Can you work these out from the drawing? Everything is in mm from the part's minimum corner. Give positions to 0.01 mm unless a question says otherwise; leave off trailing zeros. Order: outer loops, then holes, each group sorted by start corner. A loop starts at its lowest first (then second) coordinate and runs counter-clockwise, first axis right, second up. Notation, with made-up numbers: M 86.5,66.25 L 140.5,66.25 A36 cw 140.5,100.25 Z; hole C 53,9.25 d8. An arc over 180 degrees is marked long. Use a Markdown table: item, result. Add a question column.
Item 1: Suppose I cut it at B-B on z = 0.6. Count the separate pieces of the cut face and the enclosed holes in it, plus the area to 3 significant figures.
Item 2: If I drill on L1, parallel to Y at x = 25, z = 2.25; L2, parallel to Z at x = 12, y = 31.75; L3, parallel to Y at x = 17.5, z = 4.45, over which ranges is the centre line in solid material (lowest first)? Write a range as from..to.
Item 3: Suppose I cut it at A-A on y = 6. Write out the boundary of the cut face in (x, z).
Item 4: Suppose I cut it at D-D on x = 27. Write out the boundary of the cut face in (y, z), plus the area to 3 significant figures.
Item 5: Suppose I cut it at C-C on y = 13.5. Write out the boundary of the cut face in (x, z), plus the area to 3 significant figures.
Item 6: I'm going to push flat-ended pins straight in: pin 1 Ø1.5 at (x, z) = (46, 2.5) entering from -Y; pin 2 Ø0.8 at (x, z) = (46, 2.5) entering from +Y. Where does each tip first touch, or does it pass through?
Item 7: If we mould it in two halves opening along Y, with no side actions, what happens to the marked faces 1, 2 and 3? For each: released by +Y, released by -Y, zero draft, split by the parting line, or undercut.
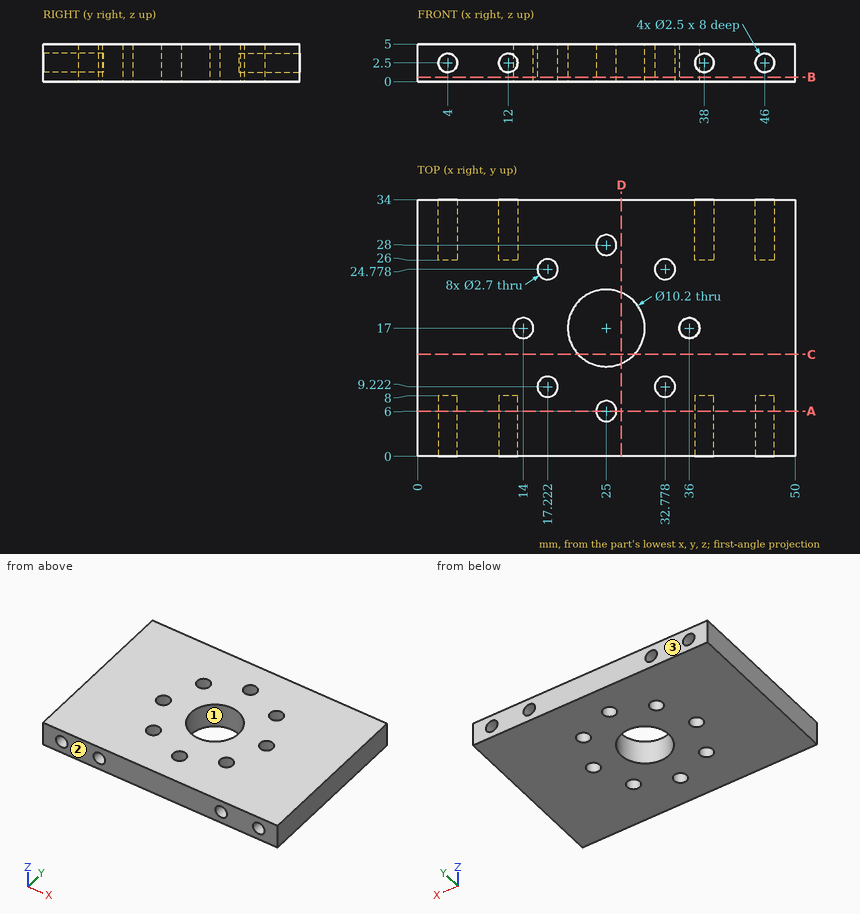
Findings below:
| question | item | result |
|---|---|---|
| 1 | separate pieces | 1 |
| 1 | enclosed holes | 9 |
| 1 | area | 1,570 mm^2 |
| 2 | L1 | y = 0..4.65, 7.35..11.9, 22.1..26.65, 29.35..34 |
| 2 | L2 | z = 0..1.25, 3.75..5 |
| 2 | L3 | y = 0..7.9, 10.54..23.46, 26.1..34 |
| 3 | outline | M 0,0 L 23.65,0 L 23.65,5 L 0,5 Z; M 26.35,0 L 50,0 L 50,5 L 26.35,5 Z; hole C 4,2.5 d2.5; hole C 12,2.5 d2.5; hole C 38,2.5 d2.5; hole C 46,2.5 d2.5 |
| 4 | outline | M 0,0 L 12.31,0 L 12.31,5 L 0,5 Z; M 21.69,0 L 34,0 L 34,5 L 21.69,5 Z |
| 4 | area | 123 mm^2 |
| 5 | outline | M 0,0 L 21.29,0 L 21.29,5 L 0,5 Z; M 28.71,0 L 50,0 L 50,5 L 28.71,5 Z |
| 5 | area | 213 mm^2 |
| 6 | pin 1 | stops at y = 8 |
| 6 | pin 2 | stops at y = 26 |
| 7 | face 1 | undercut |
| 7 | face 2 | released by -Y |
| 7 | face 3 | released by +Y |
